Work out the finished part from the listing and answer in its coordinate system (mm). Face numbers are marked on the shaded views. A direction names the side the tool comes from. Give positions to 0.01 mm unless a question says otherwise; leave off trailing zeros. Loops run counter-clockwise (first coordinate to the right, second up) from the corner with the lowest first, then second, coordinate; pieces in that order, holes last. Notation, with made-up numbers: (23.5, 80.25) - (71.5, 80.25) arc R23 cw to (71.5, 109.25) - close; hole circle Ø9 at (62, 12.5). An arc over 180 degrees is marked (long way). Use CSV: the item, a comma, the result in double quotes.
from build123d import *

# Parameters (mm, degrees)
F1_DEPTH = 1.6
F2_SCALE = 1.25


with BuildPart() as f1:
    # F0 (on Front) → F1 (new body)
    with BuildSketch(Plane.XZ):
        with BuildLine():
            Line((0, 0), (0.413425887, 0))
            Line((0.413425887, 0), (0.8268517741, 0))
            Line((0.8268517741, 0), (0.913425887, 4.9598276104))
            ThreePointArc((0.913425887, 4.9598276104), (1.0081087659, 5.1513941345), (1.2162387154, 5.1998142211))
            Line((1.2162387154, 5.1998142211), (5.5792679741, 4.2561256))
            Line((5.5792679741, 4.2561256), (4.9705727128, 5.2097686))
            ThreePointArc((4.9705727128, 5.2097686), (4.8360238518, 5.8823080691), (5.1909015741, 6.4692276))
            Line((5.1909015741, 6.4692276), (9.7032877741, 9.9448366))
            Line((9.7032877741, 9.9448366), (8.9429137741, 10.373741))
            ThreePointArc((8.9429137741, 10.373741), (8.7655752428, 10.5643141825), (8.7308237651, 10.8223053206))
            Line((8.7308237651, 10.8223053206), (9.2566129031, 13.8156465299))
            Line((9.2566129031, 13.8156465299), (6.6742096902, 13.4228908506))
            ThreePointArc((6.6742096902, 13.4228908506), (6.4203753707, 13.4717678019), (6.2541926873, 13.66976814))
            Line((6.2541926873, 13.66976814), (5.8709357741, 14.6970242))
            Line((5.8709357741, 14.6970242), (3.8084164021, 12.3209425283))
            ThreePointArc((3.8084164021, 12.3209425283), (3.1924630132, 12.2021834474), (2.9307614756, 12.7722839665))
            Line((2.9307614756, 12.7722839665), (4.1535767314, 17.8771898961))
            Line((4.1535767314, 17.8771898961), (2.8251496269, 17.1293843238))
            ThreePointArc((2.8251496269, 17.1293843238), (2.5371995805, 17.0940398171), (2.3078402562, 17.2716876815))
            Line((2.3078402562, 17.2716876815), (0.413425887, 20.5711957021))
            Line((0.413425887, 20.5711957021), (-1.4809884821, 17.2716876815))
            ThreePointArc((-1.4809884821, 17.2716876815), (-1.7103478064, 17.0940398171), (-1.9982978528, 17.1293843238))
            Line((-1.9982978528, 17.1293843238), (-3.3267249573, 17.8771898961))
            Line((-3.3267249573, 17.8771898961), (-2.1039097015, 12.7722839665))
            ThreePointArc((-2.1039097015, 12.7722839665), (-2.3656112391, 12.2021834474), (-2.9815646281, 12.3209425283))
            Line((-2.9815646281, 12.3209425283), (-5.044084, 14.6970242))
            Line((-5.044084, 14.6970242), (-5.4273409133, 13.66976814))
            ThreePointArc((-5.4273409133, 13.66976814), (-5.5935235967, 13.4717678019), (-5.8473579162, 13.4228908506))
            Line((-5.8473579162, 13.4228908506), (-8.4297611291, 13.8156465299))
            Line((-8.4297611291, 13.8156465299), (-7.903971991, 10.8223053206))
            ThreePointArc((-7.903971991, 10.8223053206), (-7.9387234687, 10.5643141825), (-8.116062, 10.373741))
            Line((-8.116062, 10.373741), (-8.876436, 9.9448366))
            Line((-8.876436, 9.9448366), (-4.3640498, 6.4692276))
            ThreePointArc((-4.3640498, 6.4692276), (-4.0091720777, 5.8823080691), (-4.1437209388, 5.2097686))
            Line((-4.1437209388, 5.2097686), (-4.7524162, 4.2561256))
            Line((-4.7524162, 4.2561256), (-0.3893869413, 5.1998142211))
            ThreePointArc((-0.3893869413, 5.1998142211), (-0.1812569918, 5.1513941345), (-0.086574113, 4.9598276104))
            Line((-0.086574113, 4.9598276104), (0, 0))
        make_face()
    extrude(amount=F1_DEPTH)


with BuildPart() as f1_1:
    # F2: moved
    add(f1.part.scale(F2_SCALE).moved(Location((-0.2067129435, 0.4, 0))))


solid = f1_1.part
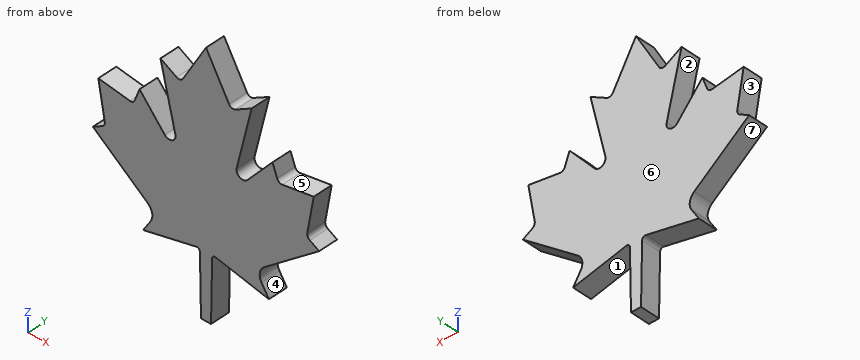
Item 1: A cutting plane is placed at A-A on z = 22. Determine the outline of the cut face in (x, y), and give its area (3 significant figures).
Determined:
outline,"(-4.28, -1.6) - (-3.75, -1.6) - (-3.75, 0.4) - (-4.28, 0.4) - close; (-1.82, -1.6) - (2.44, -1.6) - (2.44, 0.4) - (-1.82, 0.4) - close; (4.37, -1.6) - (4.9, -1.6) - (4.9, 0.4) - (4.37, 0.4) - close"
area,"10.7 mm²"
Item 2: Given P1, Ø1, axis at y = -1, z = 20.5, coming from the -X side, flat-ended and moving along its own axis, determine where the tip first touches the part or whether it passes through.
Determined:
P1,"stops at x = -4.04"
Item 3: A cutting plane is placed at B-B on x = -9.25. Determine the outline of the cut face in (y, z), and give its area (3 significant figures).
Determined:
outline,"(-1.6, 10.85) - (0.4, 10.85) - (0.4, 17.04) - (-1.6, 17.04) - close"
area,"12.4 mm²"
Item 4: Find the intervals of material crossed by line 1 (X direction, y = 0.05, z = 11.5); line 2 (Z direction, x = -2, y = -1.15); line 3 (Z direction, x = -9, y = -1.3), in increasing order.
Determined:
line 1,"x = -10.09 to 10.71"
line 2,"z = 6.22 to 21.69"
line 3,"z = 10.66 to 17"
Item 5: For the marked faces 1, 2, 3 and 4, determine the directions among +Z, -Z, +X, -X, +Y, -Y from which every point of the face is accessible in a straight line to the end or side of a thin tool.
Determined:
face 1,"-Z, +Y, -Y"
face 2,"+Y, -Y"
face 3,"-X, +Y, -Y"
face 4,"+X, +Y, -Y"
Item 6: The mould has two halves that part along X. Classify the marked faces 5, 6 and 7: pulls with the +X half, pulls with the -X half, needs draft (parallel to the pull), parting line crosses it, or undercut.
Determined:
face 5,"undercut"
face 6,"needs draft"
face 7,"pulls with the -X half"
Item 7: A cutting plane is placed at C-C on z = 11.25. Determine the outline of the cut face in (x, y), and give its area (3 significant figures).
Determined:
outline,"(-9.77, -1.6) - (10.39, -1.6) - (10.39, 0.4) - (-9.77, 0.4) - close"
area,"40.3 mm²"
